Design review of the part shown in the three views and the two pictorial views. Dimensions are in mm from the part's minimum x, y and z. A direction names the side the tool comes from. Coordinates: 2 decimals unless noted, no trailing zeros. Loops run counter-clockwise (first coordinate to the right, second up) from the corner with the lowest first, then second, coordinate; pieces in that order, holes last. Notation, with made-up numbers: (-39.5, -30.75) -> (-19.5, -30.75) arc R16 cw to (-19.5, -8.75) -> close; hole circle Ø6 at (2.5, 35). An arc over 180 degrees is marked (long way). Answer in a Markdown table with one row per item.
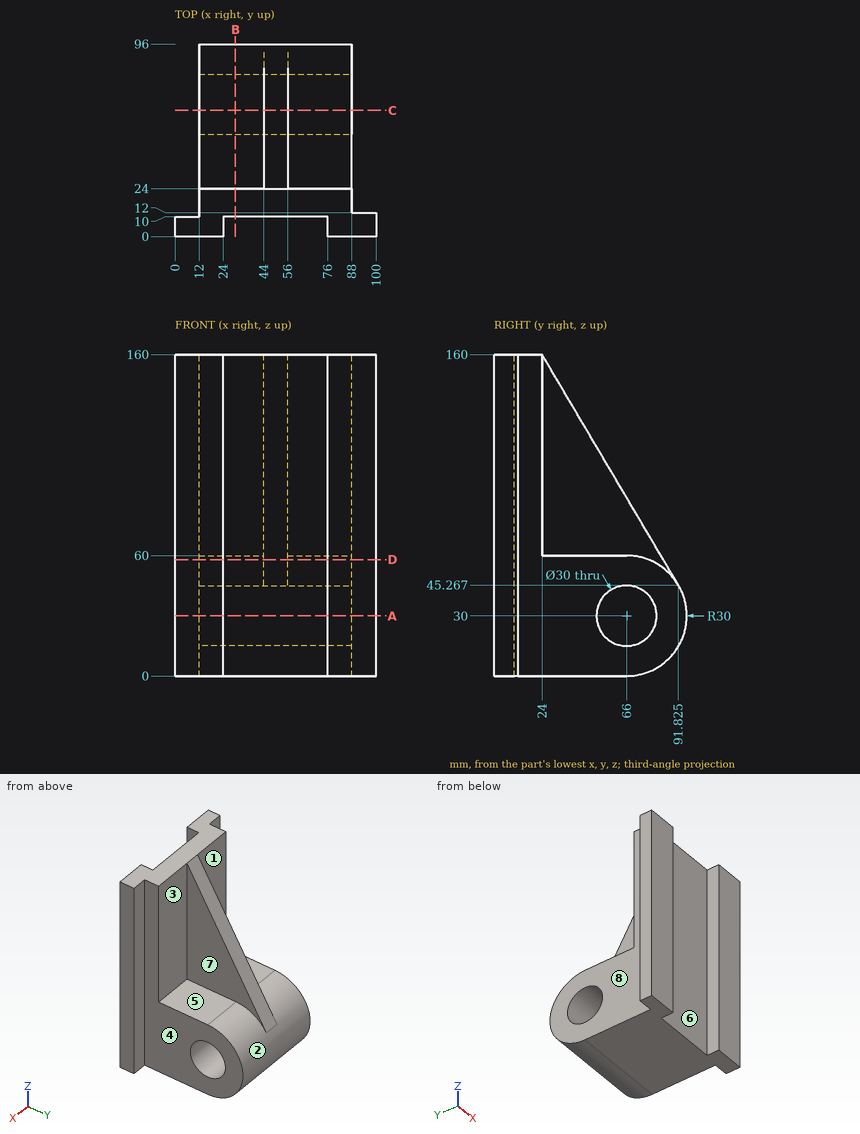
(1) Take a section at B-B on x = 30. Give the boundary of the cut face in (y, z), and give its area (3 significant figures).
Evaluation:
| item | result |
|---|---|
| outline | (10, 0) -> (66, 0) arc R30 ccw to (66, 60) -> (24, 60) -> (24, 160) -> (10, 160) -> close; hole circle Ø30 at (66, 30) |
| area | 5,470 mm² |
(2) For pin 1 (12 mm diameter, centred on x = 33.5, z = 74, fed in from +Y); pin 2 (3 mm diameter, centred on x = 21, z = 30, fed in from +Y); pin 3 (12 mm diameter, centred on x = 66, y = 56.5, fed in from +Z), all flat-tipped, find the tip position at first contact; note any pin that passes through.
Evaluation:
| item | result |
|---|---|
| pin 1 | stops at y = 24 |
| pin 2 | stops at y = 96 |
| pin 3 | stops at z = 60 |
(3) Draft analysis for pull direction X (two halves, no side actions). For the marked faces 5, 6, 7 and 8, state which applies: pulls with the +X half, pulls with the -X half, needs draft (parallel to the pull), parting line crosses it, or undercut.
Evaluation:
| item | result |
|---|---|
| face 5 | needs draft |
| face 6 | undercut |
| face 7 | pulls with the +X half |
| face 8 | pulls with the -X half |
(4) Take a section at C-C on y = 63. Give the boundary of the cut face in (x, z).
Evaluation:
| item | result |
|---|---|
| outline | (12, 0) -> (88, 0) -> (88, 15.3) -> (12, 15.3) -> close; (12, 44.7) -> (88, 44.7) -> (88, 60) -> (56, 60) -> (56, 94.03) -> (44, 94.03) -> (44, 60) -> (12, 60) -> close |
(5) To check wall thickness, follow probe 1 along Y at (x, z) = (53, 30); probe 2 along X at (y, z) = (9.5, 39); probe 3 along Z at (x, y) = (22.5, 25). State the ranges of each line that lie inside material, in increasing order.
Evaluation:
| item | result |
|---|---|
| probe 1 | y = 10 to 51, 81 to 96 |
| probe 2 | x = 0 to 24, 76 to 100 |
| probe 3 | z = 0 to 60 |
(6) Take a section at D-D on z = 58. Give the boundary of the cut face in (x, y).
Evaluation:
| item | result |
|---|---|
| outline | (0, 0) -> (24, 0) -> (24, 10) -> (76, 10) -> (76, 0) -> (100, 0) -> (100, 12) -> (88, 12) -> (88, 76.77) -> (56, 76.77) -> (56, 84.3) -> (44, 84.3) -> (44, 76.77) -> (12, 76.77) -> (12, 10) -> (0, 10) -> close |
(7) Tool access review of the marked faces 1, 2, 3 and 4: name each direction out of +Z, -Z, +X, -X, +Y, -Y from which nothing blocks a thin tool from reaching the whole face with its end or side.
Evaluation:
| item | result |
|---|---|
| face 1 | +Z, -X, +Y |
| face 2 | +Y |
| face 3 | +Z, +X, +Y |
| face 4 | +Z, -Z, +X, +Y |
(8) Take a section at A-A on z = 30. Give the boundary of the cut face in (x, y).
Evaluation:
| item | result |
|---|---|
| outline | (0, 0) -> (24, 0) -> (24, 10) -> (76, 10) -> (76, 0) -> (100, 0) -> (100, 12) -> (88, 12) -> (88, 51) -> (12, 51) -> (12, 10) -> (0, 10) -> close; (12, 81) -> (88, 81) -> (88, 96) -> (12, 96) -> close |
